Solid Edge part; units mm, degrees
sketch "Sketch1" plane through (0, 0, 0) normal (0, -1, 0) x (1, 0, 0)
  line L0 (0, 3.2) -> (6.7253, 3.2)
  line L1 (6.7253, 3.2) -> (7, 3.1)
  line L2 (7, 3.1) -> (8, 3.1)
  line L3 (8, 3.1) -> (8, 0)
  line L4 (8, 0) -> (0, 0)
  dimension "D1" = 8
  dimension "D2" = 6.7253
revolve "RevolvedProtrusion1" add sketch "Sketch1" angle 360 about axis through (0, 0, 0) along (0, 0, 1)
fillet "Round1" radius 0.5 2 edges at (-8, 0, 3.1) (-6.7253, 0, 3.2)
fillet "Round_2" radius 0.15 1 edges at (-8, 0, 0)
Geometry: final body of the model. Coordinates: model frame, mm. A direction names the side the tool comes from. Round coordinates to 2 decimals unless told otherwise and drop trailing zeros. Order: outer loops, then holes, each group sorted by start corner. A loop starts at its lowest first (then second) coordinate and runs counter-clockwise, first axis right, second up. Notation, with made-up numbers: M 72.25,87.25 L 124.25,87.25 A9 cw 124.25,103.25 Z; hole C 50,-35.75 d2. An arc over 180 degrees is marked long. One line per item, written item: value.
(1) Cut plane A-A (z = 0.45). Return the cut outline in (x, y).
Result sheet:
outline: C 0,0 d16
(2) Line query: probe 1 along Y at (x, z) = (0.25, 0.75); probe 2 along Y at (x, z) = (-3.75, 2); probe 3 along X at (y, z) = (3.5, 2.6). Output: solid intervals per line, ascending. Write a range as [from, to].
Result sheet:
probe 1: [-8, 8]
probe 2: [-7.07, 7.07]
probe 3: [-7.19, 7.19]
(3) Pin query (flat end, axial travel): P1, Ø1.5, axis at x = 3.5, z = 2.5, coming from the -Y side. Return the tip coordinate at first contact, or that it passes through.
Result sheet:
P1: y = -7.51
(4) Reachability of faces 1 (the cylindrical face through (-1.73, 7.81, 1.36)), 2 (the flat face through (7, 2, 3.1)) from +Z, -Z, +X, -X, +Y, -Y: full face, straight path, thin tool, end or side. Return the list, or none.
Result sheet:
face 1: +Z, -Z
face 2: +Z
